```python
from build123d import *

# Parameters (mm, degrees)
BOSS_EXTRUDE1_DEPTH = 360
CUT_EXTRUDE1_DEPTH  = 360
SKETCH3_R           = 8.05
BOSS_EXTRUDE2_DEPTH = 20
SKETCH4_R           = 7.873776935
BOSS_EXTRUDE3_DEPTH = 20


with BuildPart() as part:
    # Sketch1 → Boss-Extrude1 (new body)
    with BuildSketch(Plane.XY):
        Polygon((-115.5, 32.593599034), (-10, -37.406400966), (10, -37.406400966), (115.5, 32.593599034), align=None)
    extrude(amount=BOSS_EXTRUDE1_DEPTH)

    # Sketch2 → Cut-Extrude1 (cut)
    with BuildSketch(Plane.XY.offset(360)):
        Polygon((-78.867089656, 32.593599034), (82.733123463, 32.593599034), (10, -17.406400966), (-10, -17.406400966), align=None)
    extrude(amount=-CUT_EXTRUDE1_DEPTH, mode=Mode.SUBTRACT)

    # Sketch3 → Boss-Extrude2 (add)
    with BuildSketch(Plane.XY.offset(360)):
        with Locations((-0.773206761, -26.891281742)):
            Circle(SKETCH3_R)
    extrude(amount=BOSS_EXTRUDE2_DEPTH)

    # Sketch4 → Boss-Extrude3 (add)
    with BuildSketch(Plane(origin=(0, 0, 0), x_dir=(-1, 0, 0), z_dir=(0, 0, -1))):
        with Locations((0.773206761, -26.891281742)):
            Circle(SKETCH4_R)
    extrude(amount=BOSS_EXTRUDE3_DEPTH)


solid = part.part
```
Could you check a few things on this model? Use its own coordinates, in mm. A direction names the side the tool comes from. Round coordinates to 2 decimals unless told otherwise and drop trailing zeros. Loops run counter-clockwise (first coordinate to the right, second up) from the corner with the lowest first, then second, coordinate; pieces in that order, holes last. Notation, with made-up numbers: (22.25, -40) -> (66.25, -40) arc R12 cw to (66.25, -36) -> close; hole circle Ø9 at (-37.75, 31.5). An arc over 180 degrees is marked (long way). Put each result on its own line as item: value.
Q1. Please list where these lines run through material, in increasing order: line 1 (X direction, y = -9.5, z = 53); line 2 (X direction, y = -15, z = 285); line 3 (Z direction, x = -75, y = 8.5). Write a range as from..to.
Checks:
line 1: -52.06..-20.89, 21.5..52.06
line 2: -43.77..-13.31, 13.5..43.77
line 3: 0..360
Q2. I want a section at A-A on y = 6.5. Write out the boundary of the cut face in (x, z).
Checks:
outline: (-76.17, 0) -> (-42.93, 0) -> (-42.93, 360) -> (-76.17, 360) -> close; (44.78, 0) -> (76.17, 0) -> (76.17, 360) -> (44.78, 360) -> close
Q3. I want a section at C-C on x = -15. Write out the boundary of the cut face in (y, z).
Checks:
outline: (-34.09, 0) -> (-13.78, 0) -> (-13.78, 360) -> (-34.09, 360) -> close
Q4. I want a section at B-B on z = 59. Write out the boundary of the cut face in (x, y).
Checks:
outline: (-115.5, 32.59) -> (-10, -37.41) -> (10, -37.41) -> (115.5, 32.59) -> (82.73, 32.59) -> (10, -17.41) -> (-10, -17.41) -> (-78.87, 32.59) -> close
Q5. I want a section at D-D on x = -42. Write out the boundary of the cut face in (y, z).
Checks:
outline: (-16.17, 0) -> (5.83, 0) -> (5.83, 360) -> (-16.17, 360) -> close
Q6. Thinking about a two-plate mould opening in X: for faces 5 (the flat face through (-1, -27, -20)), 6 (the flat face through (62.012, -2.896, 177.48)), 7 (the flat face through (0, -17.406, 183)), 8 (the flat face through (-43.951, 7.244, 182.52)), which applies, pulls with the +X half, pulls with the -X half, needs draft (parallel to the pull), parting line crosses it, or undercut?
Checks:
face 5: needs draft
face 6: pulls with the +X half
face 7: undercut
face 8: undercut
Q7. Which directions (+Z, -Z, +X, -X, +Y, -Y) give clear straight access to the entire face, cutting with the end or side of a thin tool? Please do faces 1 (the flat face through (46.876, 7.944, 182.52)), 2 (the cylindrical face through (0.93, -34.58, -9.86)), 3 (the flat face through (-63.488, -1.916, 177.48)), 4 (the cylindrical face through (-2.52, -34.75, 369.86)).
Checks:
face 1: +Z, -Z, +Y
face 2: -Z
face 3: +Z, -Z, -X, -Y
face 4: +Z
Q8. For pin 1 Ø6 at (y, z) = (-4, 261.5) entering from +X; pin 2 Ø22 at (x, z) = (0, 210) entering from +Y; pin 3 Ø4 at (x, y) = (-58, -7) entering from +Z, each with a flat end and sliding along its axis, tell me the tip position at first contact or that it passes through.
Checks:
pin 1: x = 64.87
pin 2: y = -16.68
pin 3: z = 360
